Here's how the part is built. I have some questions about the finished solid (model axes, mm). A direction names the side the tool comes from. Round coordinates to 2 decimals unless told otherwise and drop trailing zeros. Write each loop counter-clockwise with the first axis right and the second up, starting at its lowest first coordinate (ties: lowest second). Pieces come first, ordered by that corner, then holes. Notation, with made-up numbers: (11.25, 28) -> (53.25, 28) arc R17 ccw to (53.25, 35) -> close; hole circle Ø8 at (30, 35). An arc over 180 degrees is marked (long way). Put each result on its own line as item: value. Start each with the question number.
1) I want a section at C-C, the plane z = -6.75. List the corners of the cut face in (x, y) for me.
2) I want a section at D-D, the plane z = 8.25. List the corners of the cut face in (x, y) for me, then the cut area to 3 significant figures.
3) I want a section at A-A, the plane x = -4.75. List the corners of the cut face in (y, z) for me.
4) If I drill on line 1 along X through (y, z) = (-3.25, -9); line 2 along X through (y, z) = (7.75, 1); line 3 along Y through (x, z) = (-3.25, 9.5), over which ranges is the centre line in solid material (lowest first)? Write a range as [from, to].
5) We'd pull the mould along X, two halves only. Please class faces 1 (the flat face through (0, -6.792, 0)), 2 (the flat face through (0, -6.4, 0)), 3 (the flat face through (7.978, 1, 0)): released by +X, released by -X, zero draft, split by the parting line, or undercut.
6) Which directions (+Z, -Z, +X, -X, +Y, -Y) give clear straight access to the entire face, cutting with the end or side of a thin tool? Please do faces 4 (the flat face through (-6.4, 0, 0)), 5 (the flat face through (3, 7, 12.7)), 6 (the flat face through (-2.54, 8, 5)).
7) I want a section at B-B, the plane y = -1.5. List the corners of the cut face in (x, z) for me, then the cut area to 3 significant figures.
from build123d import *

# Parameters (mm, degrees)
SKETCH1_W           = 15.95500004
SKETCH1_H           = 15.775635
SKETCH1_W_2         = 12.8
SKETCH1_H_2         = 12.8
BOSS_EXTRUDE1_DEPTH = 12.7
CUT_EXTRUDE1_DEPTH  = 12.7


with BuildPart() as part:
    # Sketch1 → Boss-Extrude1 (new body, symmetric)
    with BuildSketch(Plane.XY):
        with Locations((0, 1.0956925)):
            Rectangle(SKETCH1_W, SKETCH1_H)
        Rectangle(SKETCH1_W_2, SKETCH1_H_2, mode=Mode.SUBTRACT)
    extrude(amount=BOSS_EXTRUDE1_DEPTH, both=True)

    # Sketch2 → Cut-Extrude1 (cut)
    with BuildSketch(Plane(origin=(0, 8.98351, 0), x_dir=(1, 0, 0), z_dir=(0, 1, 0))):
        with BuildLine():
            Line((2.54, 3.175), (2.54, -12.7))
            Line((2.54, -12.7), (-2.54, -12.7))
            Line((-2.54, -12.7), (-2.54, 3.175))
            ThreePointArc((-2.54, 3.175), (0, 5.715), (2.54, 3.175))
        make_face()
    extrude(amount=-CUT_EXTRUDE1_DEPTH, mode=Mode.SUBTRACT)


solid = part.part
Findings:
1. outline: (-7.98, -6.79) -> (7.98, -6.79) -> (7.98, 8.98) -> (-7.98, 8.98) -> close; hole (-6.4, -6.4) -> (6.4, -6.4) -> (6.4, 6.4) -> (-6.4, 6.4) -> close
2. outline: (-7.98, -6.79) -> (7.98, -6.79) -> (7.98, 8.98) -> (2.54, 8.98) -> (2.54, 6.4) -> (6.4, 6.4) -> (6.4, -6.4) -> (-6.4, -6.4) -> (-6.4, 6.4) -> (-2.54, 6.4) -> (-2.54, 8.98) -> (-7.98, 8.98) -> close
2. area: 74.7 mm2
3. outline: (-6.79, -12.7) -> (-6.4, -12.7) -> (-6.4, 12.7) -> (-6.79, 12.7) -> close; (6.4, -12.7) -> (8.98, -12.7) -> (8.98, 12.7) -> (6.4, 12.7) -> close
4. line 1: x = [-7.98, -6.4], [6.4, 7.98]
4. line 2: x = [-7.98, -2.54], [2.54, 7.98]
4. line 3: y = [-6.79, -6.4], [6.4, 8.98]
5. face 1: zero draft
5. face 2: undercut
5. face 3: released by +X
6. face 4: +Z, -Z
6. face 5: +Z, +X, -X, +Y, -Y
6. face 6: +Z, +Y
7. outline: (-7.98, -12.7) -> (-6.4, -12.7) -> (-6.4, 12.7) -> (-7.98, 12.7) -> close; (6.4, -12.7) -> (7.98, -12.7) -> (7.98, 12.7) -> (6.4, 12.7) -> close
7. area: 80.1 mm2
